```python
from build123d import *

# Parameters (mm, degrees)
BOSS_EXTRUDE1_DEPTH = 9.525
BOSS_EXTRUDE2_DEPTH = 1.5875
BOSS_EXTRUDE3_DEPTH = 1.5875
BOSS_EXTRUDE4_DEPTH = 1.5875
SKETCH5_R           = 1.524
CUT_EXTRUDE1_DEPTH  = 6.08


with BuildPart() as part:
    # Sketch1 → Boss-Extrude1 (new body)
    with BuildSketch(Plane.XY):
        with BuildLine():
            Line((-1.778, -1.905), (1.778, -1.905))
            ThreePointArc((1.778, -1.905), (1.867802561, -1.867802561), (1.905, -1.778))
            Line((1.905, -1.778), (1.905, 1.778))
            ThreePointArc((1.905, 1.778), (1.867802561, 1.867802561), (1.778, 1.905))
            Line((1.778, 1.905), (-1.778, 1.905))
            ThreePointArc((-1.778, 1.905), (-1.867802561, 1.867802561), (-1.905, 1.778))
            Line((-1.905, 1.778), (-1.905, -1.778))
            ThreePointArc((-1.905, -1.778), (-1.867802561, -1.867802561), (-1.778, -1.905))
        make_face()
    extrude(amount=BOSS_EXTRUDE1_DEPTH)

    # Sketch2 → Boss-Extrude2 (add)
    with BuildSketch(Plane.XY.offset(9.525)):
        with BuildLine():
            Line((-3.048, -3.175), (3.048, -3.175))
            ThreePointArc((3.048, -3.175), (3.137802561, -3.137802561), (3.175, -3.048))
            Line((3.175, -3.048), (3.175, 3.048))
            ThreePointArc((3.175, 3.048), (3.137802561, 3.137802561), (3.048, 3.175))
            Line((3.048, 3.175), (-3.048, 3.175))
            ThreePointArc((-3.048, 3.175), (-3.137802561, 3.137802561), (-3.175, 3.048))
            Line((-3.175, 3.048), (-3.175, -3.048))
            ThreePointArc((-3.175, -3.048), (-3.137802561, -3.137802561), (-3.048, -3.175))
        make_face()
    extrude(amount=BOSS_EXTRUDE2_DEPTH)

    # Sketch3 → Boss-Extrude3 (add)
    with BuildSketch(Plane.XY.offset(11.1125)):
        with BuildLine():
            Line((-1.4605, -1.5875), (1.4605, -1.5875))
            ThreePointArc((1.4605, -1.5875), (1.550302561, -1.550302561), (1.5875, -1.4605))
            Line((1.5875, -1.4605), (1.5875, 1.4605))
            ThreePointArc((1.5875, 1.4605), (1.550302561, 1.550302561), (1.4605, 1.5875))
            Line((1.4605, 1.5875), (-1.4605, 1.5875))
            ThreePointArc((-1.4605, 1.5875), (-1.550302561, 1.550302561), (-1.5875, 1.4605))
            Line((-1.5875, 1.4605), (-1.5875, -1.4605))
            ThreePointArc((-1.5875, -1.4605), (-1.550302561, -1.550302561), (-1.4605, -1.5875))
        make_face()
    extrude(amount=BOSS_EXTRUDE3_DEPTH)

    # Sketch4 → Boss-Extrude4 (add)
    with BuildSketch(Plane.XY.offset(12.7)):
        with BuildLine():
            Line((-3.048, -3.175), (3.048, -3.175))
            ThreePointArc((3.048, -3.175), (3.137802561, -3.137802561), (3.175, -3.048))
            Line((3.175, -3.048), (3.175, 3.048))
            ThreePointArc((3.175, 3.048), (3.137802561, 3.137802561), (3.048, 3.175))
            Line((3.048, 3.175), (-3.048, 3.175))
            ThreePointArc((-3.048, 3.175), (-3.137802561, 3.137802561), (-3.175, 3.048))
            Line((-3.175, 3.048), (-3.175, -3.048))
            ThreePointArc((-3.175, -3.048), (-3.137802561, -3.137802561), (-3.048, -3.175))
        make_face()
    extrude(amount=BOSS_EXTRUDE4_DEPTH)

    # Sketch5 → Cut-Extrude1 (cut, through all)
    with BuildSketch(Plane.ZY.offset(1.905)):
        with Locations((2.2225, 0)):
            Circle(SKETCH5_R)
        with Locations((7.3025, 0)):
            Circle(SKETCH5_R)
    extrude(amount=-CUT_EXTRUDE1_DEPTH, mode=Mode.SUBTRACT)


solid = part.part
```
The model under review builds one solid part; all positions refer to its coordinate system, in mm. A direction names the side the tool comes from. Round coordinates to 2 decimals unless told otherwise and drop trailing zeros. Order: outer loops, then holes, each group sorted by start corner. A loop starts at its lowest first (then second) coordinate and runs counter-clockwise, first axis right, second up. Notation, with made-up numbers: (51, 3.5) - (73, 3.5) arc R23 ccw to (73, 15.5) - close; hole circle Ø5 at (78.5, 30). An arc over 180 degrees is marked (long way). Answer in a Markdown table with one row per item.
(1) Take a section at A-A on y = -2.5. Write out the cut boundary in (x, z) (1 decimal).
Result set:
| item | result |
|---|---|
| outline | (-3.2, 9.5) - (3.2, 9.5) - (3.2, 11.1) - (-3.2, 11.1) - close; (-3.2, 12.7) - (3.2, 12.7) - (3.2, 14.3) - (-3.2, 14.3) - close |
(2) Take a section at D-D on x = -1.25. Write out the cut boundary in (y, z) (1 decimal), plus the area to 3 significant figures.
Result set:
| item | result |
|---|---|
| outline | (-3.2, 9.5) - (-1.9, 9.5) - (-1.9, 0) - (1.9, 0) - (1.9, 9.5) - (3.2, 9.5) - (3.2, 11.1) - (1.6, 11.1) - (1.6, 12.7) - (3.2, 12.7) - (3.2, 14.3) - (-3.2, 14.3) - (-3.2, 12.7) - (-1.6, 12.7) - (-1.6, 11.1) - (-3.2, 11.1) - close; hole circle Ø3 at (0, 2.2); hole circle Ø3 at (0, 7.3) |
| area | 46.9 mm2 |
(3) Clearance check with flat-ended pins moving along their axes: P1, Ø0.8, axis at y = -0.5, z = 12, coming from the -X side; P2, Ø3, axis at x = 2, z = 6.5, coming from the +Y side (3 decimals); P3, Ø1, axis at x = -2, z = 8, coming from the -Y side (3 decimals). State where each tip first meets the part, or that it passes through.
Result set:
| item | result |
|---|---|
| P1 | stops at x = -1.59 |
| P2 | stops at y = 1.905 |
| P3 | stops at y = -1.905 |
(4) For line 1 (Y direction, x = 1.25, z = 7.25) (3 decimals); line 2 (Z direction, x = -1, y = -3) (1 decimal); line 3 (Z direction, x = 0.5, y = -0.5), list the stretches that pass through material, from the lowest coordinate up. Write a range as from..to.
Result set:
| item | result |
|---|---|
| line 1 | y = -1.905..-1.523, 1.523..1.905 |
| line 2 | z = 9.5..11.1, 12.7..14.3 |
| line 3 | z = 0..0.78, 3.66..5.86, 8.74..14.29 |
(5) Mouldability with a two-part tool opening along Z and no side actions: class faces 1 (the face through (-1.588, 0, 12)), 2 (the face through (0, 0, 14.288)), 3 (the face through (0, 0, 0)), 4 (the face through (-3.175, 0, 10)) as released by +Z, released by -Z, zero draft, split by the parting line, or undercut.
Result set:
| item | result |
|---|---|
| face 1 | undercut |
| face 2 | released by +Z |
| face 3 | released by -Z |
| face 4 | zero draft |
(6) Take a section at C-C on y = 0. Write out the cut boundary in (x, z) (1 decimal), plus the area to 3 significant figures.
Result set:
| item | result |
|---|---|
| outline | (-3.2, 9.5) - (-1.9, 9.5) - (-1.9, 8.8) - (1.9, 8.8) - (1.9, 9.5) - (3.2, 9.5) - (3.2, 11.1) - (1.6, 11.1) - (1.6, 12.7) - (3.2, 12.7) - (3.2, 14.3) - (-3.2, 14.3) - (-3.2, 12.7) - (-1.6, 12.7) - (-1.6, 11.1) - (-3.2, 11.1) - close; (-1.9, 0) - (1.9, 0) - (1.9, 0.7) - (-1.9, 0.7) - close; (-1.9, 3.7) - (1.9, 3.7) - (1.9, 5.8) - (-1.9, 5.8) - close |
| area | 38.3 mm2 |
(7) Machinability: for faces 5 (the face through (1.588, 0, 12)), 6 (the face through (0, 1.588, 12)), 7 (the face through (0, -1.588, 12)), 8 (the face through (2, 0, 12.7)), 9 (the face through (-1.905, 0, 5)), which of the approach directions +Z, -Z, +X, -X, +Y, -Y give a long, thin tool a straight path to every point of the face, cutting with its end or side? Answer none if there is none.
Result set:
| item | result |
|---|---|
| face 5 | +X, +Y, -Y |
| face 6 | +X, -X, +Y |
| face 7 | +X, -X, -Y |
| face 8 | none |
| face 9 | -Z, -X, +Y, -Y |
